Geometry: see drawing. Coordinates: mm, zero at the bounding-box minimum. A direction names the side the tool comes from. Coordinates: 2 decimals unless noted, no trailing zeros. Loops run counter-clockwise (first coordinate to the right, second up) from the corner with the lowest first, then second, coordinate; pieces in that order, holes last.
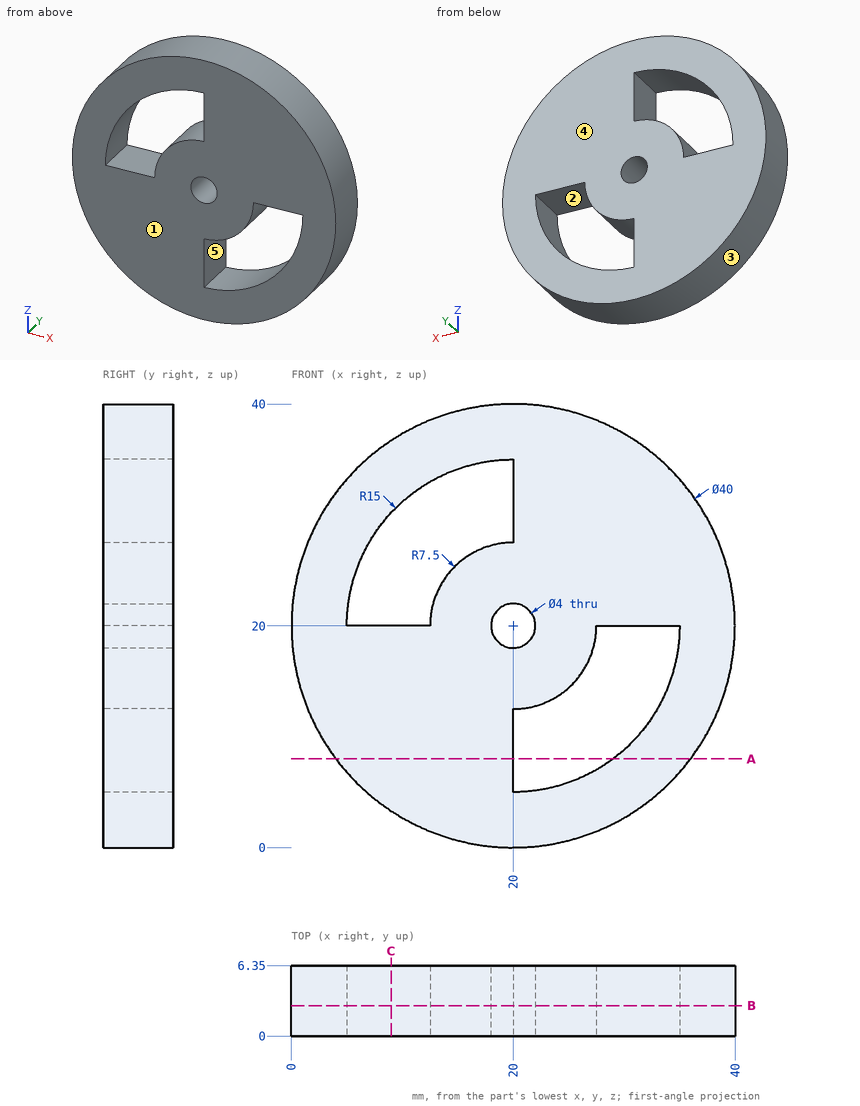
Item 1: Line query: L1, parallel to X at y = 3, z = 19 (1 decimal); L2, parallel to X at y = 3.75, z = 19.5; L3, parallel to Z at x = 21, y = 4.25 (1 decimal). Output: solid intervals per line, ascending.
Result:
L1: x = 0 to 18.3, 21.7 to 27.4, 35 to 40
L2: x = 0.01 to 18.06, 21.94 to 27.48, 34.99 to 39.99
L3: z = 0 to 5, 12.6 to 18.3, 21.7 to 40
Item 2: Contact query for flat-ended pins moving along their axis: P1, Ø3, axis at y = 4, z = 7, coming from the +X side; P2, Ø2, axis at y = 3.5, z = 10.5, coming from the -X side; P3, Ø2, axis at x = 13, y = 3, coming from the -Z side. Output: stop coordinate, or through.
Result:
P1: stops at x = 36.36
P2: stops at x = 1.9
P3: stops at z = 0.92
Item 3: Section query C-C (x = 9). Output: boundary loops of the cut face in (y, z).
Result:
outline: (0, 3.3) - (6.35, 3.3) - (6.35, 20) - (0, 20) - close; (0, 30.2) - (6.35, 30.2) - (6.35, 36.7) - (0, 36.7) - close
Item 4: Section query B-B (y = 2.75). Output: boundary loops of the cut face in (x, z), then the cut area to 3 significant figures.
Result:
outline: circle Ø40 at (20, 20); hole (5, 20) - (12.5, 20) arc R7.5 cw to (20, 27.5) - (20, 35) arc R15 ccw to start; hole circle Ø4 at (20, 20); hole (20, 5) arc R15 ccw to (35, 20) - (27.5, 20) arc R7.5 cw to (20, 12.5) - close
area: 979 mm2
Item 5: Reachability of the marked faces 4 and 5 from +Z, -Z, +X, -X, +Y, -Y: full face, straight path, thin tool, end or side. Return the list, or none.
Result:
face 4: +Z, -Z, +X, -X, +Y
face 5: +Y, -Y
Item 6: Section query A-A (z = 8). Output: boundary loops of the cut face in (x, y), then the cut area to 3 significant figures.
Result:
outline: (4, 0) - (20, 0) - (20, 6.35) - (4, 6.35) - close; (29, 0) - (36, 0) - (36, 6.35) - (29, 6.35) - close
area: 146 mm2
Item 7: Mould query, pull axis X, two halves, no side actions, for the marked faces 1, 2 and 3. Classes: +X half, -X half, draft (parallel to the pull), parting line (faces both ways), or undercut.
Result:
face 1: draft
face 2: undercut
face 3: parting line
